The drawing under review shows one solid part. Ordinate dimensions are in mm from its lowest x, y, z. Coordinates: 2 decimals unless noted, no trailing zeros. Loops run counter-clockwise (first coordinate to the right, second up) from the corner with the lowest first, then second, coordinate; pieces in that order, holes last. Notation, with made-up numbers: M -37.5,84 L 20.5,84 A25 cw 20.5,112 Z; hole C 84,-17.75 d10. An arc over 180 degrees is marked long. Answer as CSV lines item,"result". Start each with the question number.
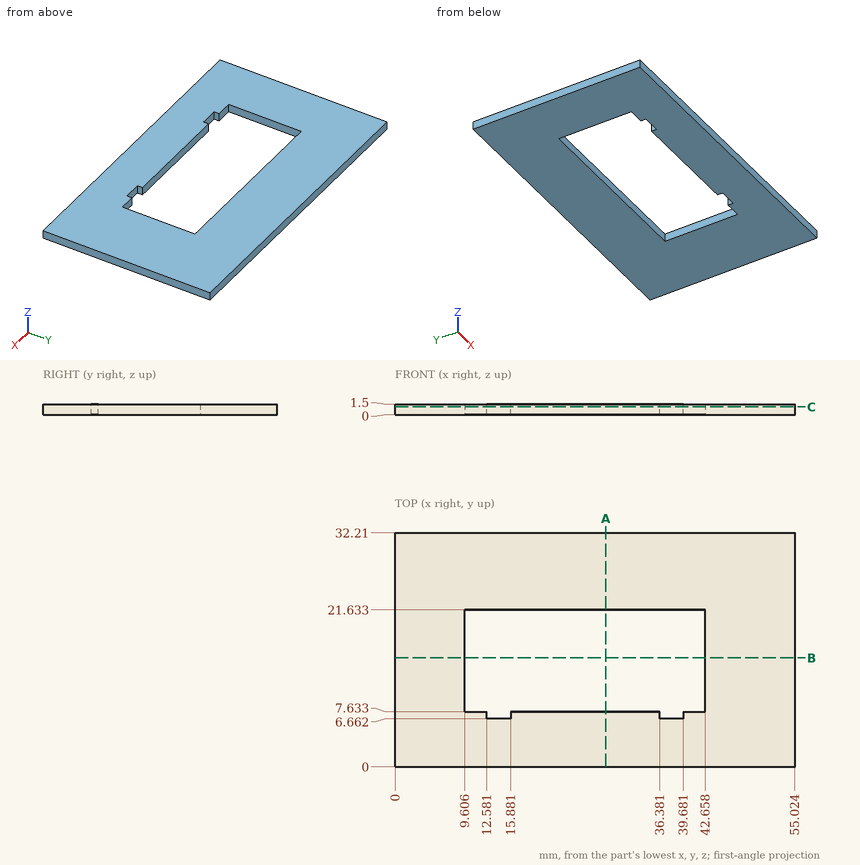
Item 1: Add section B-B (y = 15). Give the boundary of the cut face in (x, z).
Item 2: Add section A-A (x = 29). Give the boundary of the cut face in (y, z).
Item 3: Add section C-C (z = 1.1). Give the boundary of the cut face in (x, y).
Item 4: For line 1 along X through (y, z) = (7.5, 0.75); line 2 along X through (y, z) = (18.5, 0.3); line 3 along Y through (x, z) = (36, 0.9), list the stretches that pass through material, from the lowest coordinate up. Write a range as from..to.
Response:
1,outline,"M 0,0 L 9.61,0 L 9.61,1.5 L 0,1.5 Z; M 42.66,0 L 55.02,0 L 55.02,1.5 L 42.66,1.5 Z"
2,outline,"M 0,0 L 7.63,0 L 7.63,1.5 L 0,1.5 Z; M 21.63,0 L 32.21,0 L 32.21,1.5 L 21.63,1.5 Z"
3,outline,"M 0,0 L 55.02,0 L 55.02,32.21 L 0,32.21 Z; hole M 9.61,7.63 L 12.58,7.63 L 12.58,6.66 L 15.88,6.66 L 15.88,7.63 L 36.38,7.63 L 36.38,6.66 L 39.68,6.66 L 39.68,7.63 L 42.66,7.63 L 42.66,21.63 L 9.61,21.63 Z"
4,line 1,"0..12.58, 15.88..36.38, 39.68..55.02"
4,line 2,"0..9.61, 42.66..55.02"
4,line 3,"0..7.63, 21.63..32.21"
